from build123d import *

# Parameters (mm, degrees)
EXTRUDE_1_DEPTH     = 18
SKETCH_2_R          = 1.75
CUT_EXTRUDE_1_DEPTH = 13
SKETCH_3_W          = 18
SKETCH_3_H          = 10
EXTRUDE_2_DEPTH     = 4
SKETCH_10_R         = 1.75
CUT_EXTRUDE_2_DEPTH = 49.825569575
FILLET_1_R          = 10


with BuildPart() as part:
    # 草图1 → 凸台-拉伸1 (new body)
    with BuildSketch(Plane.XY):
        Polygon((0, 0), (4, 0), (4, 28.432425182), (24.819457366, 35.999089204), (24.819457366, 37.999089204), (0, 35), align=None)
    extrude(amount=EXTRUDE_1_DEPTH)

    # 草图2 → 切除-拉伸1 (cut)
    with BuildSketch(Plane.ZY):
        with Locations(Location((11.5, 5, 0), (0, 0, 270))):
            Circle(SKETCH_2_R)
    extrude(amount=-CUT_EXTRUDE_1_DEPTH, mode=Mode.SUBTRACT)

    # 草图3 → 凸台-拉伸2 (add)
    with BuildSketch(Plane.XY.offset(18)):
        with Locations((9, 5)):
            Rectangle(SKETCH_3_W, SKETCH_3_H)
    extrude(amount=EXTRUDE_2_DEPTH)

    # 草图10 → 切除-拉伸2 (cut, through all)
    with BuildSketch(Plane(origin=(0, 0, 18), x_dir=(-1, 0, 0), z_dir=(0, 0, -1))):
        with Locations((-10.5, 5)):
            Circle(SKETCH_10_R)
    extrude(amount=-CUT_EXTRUDE_2_DEPTH, mode=Mode.SUBTRACT)

    # 圆角1
    # the kernel refuses this fillet: 10 mm, written as the material it adds along each edge
    with BuildSketch(Plane(origin=(4, 10, 18), x_dir=(0, 1, 0), z_dir=(-1, 0, 0))) as fillet_1_piece_1:
        with BuildLine():
            CenterArc((8, -10), FILLET_1_R, 90, 53.130102354)
            Line((0, -4), (0, 0))
            Line((0, 0), (8, 0))
        make_face()
    extrude(amount=4)


solid = part.part
Input: part model. Units: mm. Frame: model coordinates. A direction names the side the tool comes from. Coordinates: 2 decimals unless noted, no trailing zeros. Loops run counter-clockwise (first coordinate to the right, second up) from the corner with the lowest first, then second, coordinate; pieces in that order, holes last.
(1) Section D-D on x = 10.5. Return the cut outline in (y, z).
(2) Section A-A on z = 11.5. Return the cut outline in (x, y), then the cut area to 3 significant figures.
(3) Section C-C on x = 6.25. Return the cut outline in (y, z).
(4) First-contact query: pin 1 Ø2 at (x, z) = (12.5, 20.5) entering from +Y; pin 2 Ø3 at (y, z) = (6, 20.5) entering from +X; pin 3 Ø11 at (x, y) = (11, 6.5) entering from -Z. Flat tips, straight axial feed; report the tip coordinate or a pass-through.
(5) Material intervals for probe 1 along Y at (x, z) = (10.5, 20.95); probe 2 along X at (y, z) = (14.5, 16.25); probe 3 along Z at (x, y) = (1, 23), sorted ascending.
(6) Section B-B on y = 5. Return the cut outline in (x, z).
(7) Set-up query: faces 5 (the face through (7, 30, 18)), 6 (the face through (12.58, 36.52, 8.87)), 7 (the face through (11, 10, 20)). Return all of +Z, -Z, +X, -X, +Y, -Y with unobstructed straight access to the full face (end or side cutting, diameter ignored); none if empty.
(8) Pull-direction query (Z, two-part tool) for faces 1 (the face through (2.028, 13.586, 19.027)), 2 (the face through (24.819, 37, 9)), 3 (the face through (1.972, 5.228, 13.235)), 4 (the face through (12.5, 5.1, 18)); classes: released by +Z, released by -Z, zero draft, split by the parting line, or undercut.
Data:
1. outline: (0, 18) - (3.25, 18) - (3.25, 22) - (0, 22) - close; (6.75, 18) - (10, 18) - (10, 22) - (6.75, 22) - close; (30.79, 0) - (36.27, 0) - (36.27, 18) - (30.79, 18) - close
2. outline: (0, 0) - (4, 0) - (4, 3.25) - (0, 3.25) - close; (0, 6.75) - (4, 6.75) - (4, 28.43) - (24.82, 36) - (24.82, 38) - (0, 35) - close
2. area: 221 mm2
3. outline: (0, 18) - (10, 18) - (10, 22) - (0, 22) - close; (29.25, 0) - (35.76, 0) - (35.76, 18) - (29.25, 18) - close
4. pin 1: stops at y = 10
4. pin 2: stops at x = 18
4. pin 3: stops at z = 18
5. probe 1: y = 0 to 3.25, 6.75 to 10
5. probe 2: x = 0 to 4
5. probe 3: z = 0 to 18
6. outline: (0, 0) - (4, 0) - (4, 9.75) - (0, 9.75) - close; (0, 13.25) - (4, 13.25) - (4, 18) - (8.75, 18) - (8.75, 22) - (0, 22) - close; (12.25, 18) - (18, 18) - (18, 22) - (12.25, 22) - close
7. face 5: +Z, +X, -X, +Y
7. face 6: +Z, -Z, -X, +Y
7. face 7: +Z, -Z, +X, +Y
8. face 1: released by +Z
8. face 2: zero draft
8. face 3: undercut
8. face 4: released by -Z
